```python
from build123d import *

# Parameters (mm, degrees)
EXTRUDE_THIN2_DEPTH  = 200
CUT_EXTRUDE2_REACH   = 285.304
SKETCH6_R            = 1.5
LPATTERN1_COUNT      = 8
LPATTERN1_PITCH      = 5
LPATTERN1_COUNT_DIR2 = 8
LPATTERN1_PITCH_DIR2 = 22.5
CUT_EXTRUDE3_REACH   = 286.366
SKETCH7_R            = 1.5
LPATTERN2_COUNT      = 4
LPATTERN2_PITCH      = 64
CUT_EXTRUDE4_REACH   = 281.713
SKETCH8_R            = 1.5
SKETCH8_W            = 165
SKETCH8_H            = 106
BOSS_EXTRUDE1_DEPTH  = 200
SKETCH10_W           = 200
SKETCH10_H           = 3.535533906
BOSS_EXTRUDE2_DEPTH  = 20
CUT_EXTRUDE5_REACH   = 300.814
SKETCH11_R           = 2
LPATTERN3_COUNT      = 4
LPATTERN3_PITCH      = 60
BOSS_EXTRUDE3_DEPTH  = 3
CUT_EXTRUDE6_REACH   = 299.061
SKETCH13_R           = 1.5
LPATTERN4_COUNT      = 3
LPATTERN4_PITCH      = 63.5
LPATTERN4_COUNT_DIR2 = 2
LPATTERN4_PITCH_DIR2 = 197
SKETCH16_W           = 3
SKETCH16_H           = 10
BOSS_EXTRUDE4_DEPTH  = 10
CUT_EXTRUDE7_REACH   = 299.061
SKETCH17_R           = 1.5


with BuildPart() as part:
    # Sketch4 → Extrude-Thin2 (new body)
    with BuildSketch(Plane(origin=(0, 0, 0), x_dir=(0, 0, -1), z_dir=(1, 0, 0))):
        Polygon((0, 0), (-8, 0), (-8, 3), (-72, 3), (-170.994949366, 101.994949366), (-174.530483272, 98.45941546), (-74.071067812, -2), (-13, -2), (-13, -5), (0, -5), align=None)
    extrude(amount=EXTRUDE_THIN2_DEPTH)

    # Sketch6 → Cut-Extrude2 (cut, up to next)
    with BuildSketch(Plane(origin=(0, 3, 0), x_dir=(1, 0, 0), z_dir=(0, 1, 0)), mode=Mode.PRIVATE) as cut_extrude2_sk1:
        with Locations(Location((178.75, -16, 0), (0, 0, 270))):
            Circle(SKETCH6_R)
    cut_extrude2_tool1 = extrude(cut_extrude2_sk1.sketch, amount=-CUT_EXTRUDE2_REACH, mode=Mode.PRIVATE) & part.part
    cut_extrude2 = cut_extrude2_tool1.solids().sort_by_distance((178.75, 3, 16))[0]
    add(cut_extrude2, mode=Mode.SUBTRACT)

    # LPattern1: Cut-Extrude2 8 × 8
    with Locations(*[(-j * LPATTERN1_PITCH_DIR2, 0, i * LPATTERN1_PITCH) for i in range(LPATTERN1_COUNT) for j in range(LPATTERN1_COUNT_DIR2) if (i, j) != (0, 0)]):
        add(cut_extrude2, mode=Mode.SUBTRACT)

    # Sketch7 → Cut-Extrude3 (cut, up to next)
    with BuildSketch(Plane(origin=(0, 0, 0), x_dir=(1, 0, 0), z_dir=(0, 1, 0)), mode=Mode.PRIVATE) as cut_extrude3_sk1:
        with Locations(Location((196, -4, 0), (0, 0, 270))):
            Circle(SKETCH7_R)
    cut_extrude3_tool1 = extrude(cut_extrude3_sk1.sketch, amount=-CUT_EXTRUDE3_REACH, mode=Mode.PRIVATE) & part.part
    cut_extrude3 = cut_extrude3_tool1.solids().sort_by_distance((196, 0, 4))[0]
    add(cut_extrude3, mode=Mode.SUBTRACT)

    # LPattern2: Cut-Extrude3 ×4
    with Locations(*[(-i * LPATTERN2_PITCH, 0, 0) for i in range(1, LPATTERN2_COUNT)]):
        add(cut_extrude3, mode=Mode.SUBTRACT)

    # Sketch8 → Cut-Extrude4 (cut, up to next)
    with BuildSketch(Plane(origin=(0, -34.5, 34.5), x_dir=(1, 0, 0), z_dir=(0, 0.7071067811865465, -0.7071067811865486)), mode=Mode.PRIVATE) as cut_extrude4_sk1:
        with Locations(Location((19, -180.533008589, 0), (0, 0, 270))):
            Circle(SKETCH8_R)
    cut_extrude4_tool1 = extrude(cut_extrude4_sk1.sketch, amount=-CUT_EXTRUDE4_REACH, mode=Mode.PRIVATE) & part.part
    # Sketch8 → Cut-Extrude4 (cut, up to next)
    with BuildSketch(Plane(origin=(0, -34.5, 34.5), x_dir=(1, 0, 0), z_dir=(0, 0.7071067811865465, -0.7071067811865486)), mode=Mode.PRIVATE) as cut_extrude4_sk2:
        with Locations(Location((19, -65.533008589, 0), (0, 0, 270))):
            Circle(SKETCH8_R)
    cut_extrude4_tool2 = extrude(cut_extrude4_sk2.sketch, amount=-CUT_EXTRUDE4_REACH, mode=Mode.PRIVATE) & part.part
    # Sketch8 → Cut-Extrude4 (cut, up to next)
    with BuildSketch(Plane(origin=(0, -34.5, 34.5), x_dir=(1, 0, 0), z_dir=(0, 0.7071067811865465, -0.7071067811865486)), mode=Mode.PRIVATE) as cut_extrude4_sk3:
        with Locations(Location((181, -65.533008589, 0), (0, 0, 270))):
            Circle(SKETCH8_R)
    cut_extrude4_tool3 = extrude(cut_extrude4_sk3.sketch, amount=-CUT_EXTRUDE4_REACH, mode=Mode.PRIVATE) & part.part
    # Sketch8 → Cut-Extrude4 (cut, up to next)
    with BuildSketch(Plane(origin=(0, -34.5, 34.5), x_dir=(1, 0, 0), z_dir=(0, 0.7071067811865465, -0.7071067811865486)), mode=Mode.PRIVATE) as cut_extrude4_sk4:
        with Locations(Location((181, -180.533008589, 0), (0, 0, 270))):
            Circle(SKETCH8_R)
    cut_extrude4_tool4 = extrude(cut_extrude4_sk4.sketch, amount=-CUT_EXTRUDE4_REACH, mode=Mode.PRIVATE) & part.part
    # Sketch8 → Cut-Extrude4 (cut, up to next)
    with BuildSketch(Plane(origin=(0, -34.5, 34.5), x_dir=(1, 0, 0), z_dir=(0, 0.7071067811865465, -0.7071067811865486)), mode=Mode.PRIVATE) as cut_extrude4_sk5:
        with Locations((100, -123.033008589)):
            Rectangle(SKETCH8_W, SKETCH8_H)
    cut_extrude4_tool5 = extrude(cut_extrude4_sk5.sketch, amount=-CUT_EXTRUDE4_REACH, mode=Mode.PRIVATE) & part.part
    add(cut_extrude4_tool1.solids().sort_by_distance((19, 93.156115, 162.156115))[0], mode=Mode.SUBTRACT)
    add(cut_extrude4_tool2.solids().sort_by_distance((19, 11.838835, 80.838835))[0], mode=Mode.SUBTRACT)
    add(cut_extrude4_tool3.solids().sort_by_distance((181, 11.838835, 80.838835))[0], mode=Mode.SUBTRACT)
    add(cut_extrude4_tool4.solids().sort_by_distance((181, 93.156115, 162.156115))[0], mode=Mode.SUBTRACT)
    add(cut_extrude4_tool5.solids().sort_by_distance((100, 52.497475, 121.497475))[0], mode=Mode.SUBTRACT)

    # Sketch9 → Boss-Extrude1 (add)
    with BuildSketch(Plane(origin=(200, 0, 0), x_dir=(0, 0, -1), z_dir=(1, 0, 0))):
        Polygon((-170.994949366, 101.994949366), (-174.530483272, 101.994949366), (-174.530483272, 98.45941546), align=None)
    extrude(amount=-BOSS_EXTRUDE1_DEPTH)

    # Sketch10 → Boss-Extrude2 (add)
    with BuildSketch(Plane.XY.offset(174.530483272)):
        with Locations((100, 100.227182413)):
            Rectangle(SKETCH10_W, SKETCH10_H)
    extrude(amount=BOSS_EXTRUDE2_DEPTH)

    # Sketch11 → Cut-Extrude5 (cut, up to next)
    with BuildSketch(Plane(origin=(0, 101.994949366, 0), x_dir=(1, 0, 0), z_dir=(0, 1, 0)), mode=Mode.PRIVATE) as cut_extrude5_sk1:
        with Locations(Location((190, -184.530483272, 0), (0, 0, 270))):
            Circle(SKETCH11_R)
    cut_extrude5_tool1 = extrude(cut_extrude5_sk1.sketch, amount=-CUT_EXTRUDE5_REACH, mode=Mode.PRIVATE) & part.part
    cut_extrude5 = cut_extrude5_tool1.solids().sort_by_distance((190, 101.994949, 184.530483))[0]
    add(cut_extrude5, mode=Mode.SUBTRACT)

    # LPattern3: Cut-Extrude5 ×4
    with Locations(*[(-i * LPATTERN3_PITCH, 0, 0) for i in range(1, LPATTERN3_COUNT)]):
        add(cut_extrude5, mode=Mode.SUBTRACT)

    # Sketch12 → Boss-Extrude3 (add)
    with BuildSketch(Plane(origin=(200, 0, 0), x_dir=(0, 0, -1), z_dir=(1, 0, 0))):
        Polygon((-174.530483272, 98.45941546), (-174.530483272, 87.852813742), (-163.923881554, 87.852813742), align=None)
    boss_extrude3 = extrude(amount=-BOSS_EXTRUDE3_DEPTH)

    # Sketch13 → Cut-Extrude6 (cut, up to next)
    with BuildSketch(Plane(origin=(200, 0, 0), x_dir=(0, 0, -1), z_dir=(1, 0, 0)), mode=Mode.PRIVATE) as cut_extrude6_sk1:
        with Locations((-170.530483272, 91.852813742)):
            Circle(SKETCH13_R)
    cut_extrude6_tool1 = extrude(cut_extrude6_sk1.sketch, amount=-CUT_EXTRUDE6_REACH, mode=Mode.PRIVATE) & part.part
    cut_extrude6 = cut_extrude6_tool1.solids().sort_by_distance((200, 91.852814, 170.530483))[0]
    add(cut_extrude6, mode=Mode.SUBTRACT)

    # LPattern4: Boss-Extrude3, Cut-Extrude6 3 × 2
    with Locations(*[Vector(0, -0.7071067811865724, -0.7071067811865227) * (i * LPATTERN4_PITCH) + Vector(-1, 0, 0) * (j * LPATTERN4_PITCH_DIR2) for i in range(LPATTERN4_COUNT) for j in range(LPATTERN4_COUNT_DIR2) if (i, j) != (0, 0)]):
        add(boss_extrude3)
        add(cut_extrude6, mode=Mode.SUBTRACT)

    # Sketch16 → Boss-Extrude4 (add)
    with BuildSketch(Plane.XZ.offset(2)):
        with Locations((198.5, 43.536067812)):
            Rectangle(SKETCH16_W, SKETCH16_H)
    extrude(amount=BOSS_EXTRUDE4_DEPTH)

    # Sketch17 → Cut-Extrude7 (cut, up to next)
    with BuildSketch(Plane(origin=(200, 0, 0), x_dir=(0, 0, -1), z_dir=(1, 0, 0)), mode=Mode.PRIVATE) as cut_extrude7_sk1:
        with Locations((-43.536067812, -7)):
            Circle(SKETCH17_R)
    cut_extrude7_tool1 = extrude(cut_extrude7_sk1.sketch, amount=-CUT_EXTRUDE7_REACH, mode=Mode.PRIVATE) & part.part
    add(cut_extrude7_tool1.solids().sort_by_distance((200, -7, 43.536068))[0], mode=Mode.SUBTRACT)


solid = part.part
```
The listing builds one solid part. Answer for the finished solid, in the listing's coordinates (mm). A direction names the side the tool comes from. Give positions to 0.01 mm unless a question says otherwise; leave off trailing zeros. Order: outer loops, then holes, each group sorted by start corner. A loop starts at its lowest first (then second) coordinate and runs counter-clockwise, first axis right, second up. Notation, with made-up numbers: (70, 59) - (85, 59) arc R22 cw to (85, 66) - close; hole circle Ø11 at (26.5, 58). An arc over 180 degrees is marked (long way). Answer in a Markdown table with one row per item. Add a question column.
Q1. Which of the six approach directions +Z, -Z, +X, -X, +Y, -Y give full straight-line access (tool end or side, diameter ignored) to faces 4 (the flat face through (99, 98.459, 184)), 5 (the flat face through (99, 3, 40)), 6 (the flat face through (197, 90, 172)), 7 (the flat face through (197, -6, 42))?
Q2. Find the intervals of material crossed by line 1 along Y through (x, z) = (11.5, 15); line 2 along Y through (x, z) = (31, 12.5); line 3 along Z through (x, y) = (10, 101.3), in increasing order. Write a range as [from, to].
Q3. The part is cut by section C-C (z = 96.5). Determine the outline of the cut face in (x, y).
Q4. Given P1, Ø6, axis at x = 161.5, z = 80.5, coming from the -Y side; P2, Ø3.5, axis at x = 156.25, z = 21, coming from the +Y side; P3, Ø4, axis at x = 178.75, z = 41, coming from the -Y side; P4, Ø5, axis at y = 2.05, z = 80.73, coming from the -X side, each flat-ended and moving along its own axis, determine where each tip first touches the part or whether it passes through.
Q5. The part is cut by section B-B (y = 30.5). Determine the outline of the cut face in (x, z).
Q6. For a pull along Y with two mould halves and no side action, classify faces 1 (the flat face through (3, 90, 172)), 2 (the flat face through (99, 0, 4)), 3 (the cylindrical face through (19.451, 92.425, 164.911)) as released by +Y, released by -Y, zero draft, split by the parting line, or undercut.
Q7. The part is cut by section A-A (x = 174.5). Determine the outline of the cut face in (y, z), then the cut area to 3 significant figures.
Determined:
| question | item | result |
|---|---|---|
| 1 | face 4 | +Z, +X, -X, -Y |
| 1 | face 5 | -Z, +X, -X, +Y |
| 1 | face 6 | +Z, -Y |
| 1 | face 7 | +Z, -X, -Y |
| 2 | line 1 | y = [-2, 3] |
| 2 | line 2 | y = [-5, 3] |
| 2 | line 3 | z = [170.3, 182.53], [186.53, 194.53] |
| 3 | outline | (0, 20.43) - (17.5, 20.43) - (17.5, 27.5) - (0, 27.5) - close; (182.5, 20.43) - (200, 20.43) - (200, 27.5) - (182.5, 27.5) - close |
| 4 | P1 | stops at y = 1.43 |
| 4 | P2 | stops at y = 3 |
| 4 | P3 | stops at y = -2 |
| 4 | P4 | stops at x = 0 |
| 5 | outline | (0, 99.5) - (17.5, 99.5) - (17.5, 106.57) - (0, 106.57) - close; (182.5, 99.5) - (200, 99.5) - (200, 106.57) - (182.5, 106.57) - close |
| 6 | face 1 | zero draft |
| 6 | face 2 | released by +Y |
| 6 | face 3 | undercut |
| 7 | outline | (-5, 0) - (0, 0) - (0, 8) - (3, 8) - (3, 72) - (15.02, 84.02) - (11.49, 87.56) - (-2, 74.07) - (-2, 13) - (-5, 13) - close; (86.44, 162.51) - (89.97, 158.97) - (101.99, 170.99) - (101.99, 194.53) - (98.46, 194.53) - (98.46, 174.53) - close |
| 7 | area | 632 mm² |
